from build123d import *

# Parameters (mm, degrees)
F1_W         = 60.96
F1_H         = 78.5
F2_DEPTH     = 21.5
F0_W         = 55.88
F0_H         = 73.5
F3_DEPTH     = 19.5
F4_W         = 78.5
F4_H         = 3
F5_DEPTH     = 2.54
F6_W         = 78.5
F6_H         = 3
F7_DEPTH     = 2.54
F8_W         = 44.0962035209
F8_H         = 7.4383728206
F9_DEPTH     = 2.5
F10_W        = 5.08
F10_H        = 21.59
F11_DEPTH    = 25.4
F12_R        = 1.27
F13_R        = 1.27
F14_DEPTH    = 101.6
F15_R        = 1.27
F16_DEPTH    = 25.4
F17_T1_DEPTH = 2.54
F18_F1_R     = 5.08
F18_T2_DEPTH = 103.9


# Not quite as in the source:
# - a fillet or chamfer that OpenCascade refuses, or shapes differently, is made with other operations: its cross-section is extruded or revolved along the edge and cut away or added


with BuildPart() as f2:
    # F1 (on Top) → F2 (new body)
    with BuildSketch(Plane.XY):
        with Locations((27.94, 36.75)):
            Rectangle(F1_W, F1_H)
    extrude(amount=F2_DEPTH)

    # F0 (on Top) → F3 (cut)
    with BuildSketch(Plane.XY):
        with Locations((27.94, 36.75)):
            Rectangle(F0_W, F0_H)
    extrude(amount=F3_DEPTH, mode=Mode.SUBTRACT)

    # F4 (on face) → F5 (join, through all)
    with BuildSketch(Plane.YZ.offset(58.42)):
        with Locations((36.75, -1.5)):
            Rectangle(F4_W, F4_H)
    extrude(amount=-F5_DEPTH)

    # F6 (on face) → F7 (join, through all)
    with BuildSketch(Plane(origin=(-2.54, 0, 0), x_dir=(0, -1, 0), z_dir=(-1, 0, 0))):
        with Locations((-36.75, -1.5)):
            Rectangle(F6_W, F6_H)
    extrude(amount=-F7_DEPTH)

    # F8 (on face) → F9 (join, through all)
    with BuildSketch(Plane.XZ.offset(2.5)):
        with Locations((27.1060718223, 8.4709739313)):
            Rectangle(F8_W, F8_H)
    extrude(amount=-F9_DEPTH)

    # F10 (on face) → F11 (cut)
    with BuildSketch(Plane(origin=(-2.54, 0, 0), x_dir=(0, -1, 0), z_dir=(-1, 0, 0))):
        with Locations((-2.54, 7.795)):
            Rectangle(F10_W, F10_H)
    extrude(amount=-F11_DEPTH, mode=Mode.SUBTRACT)

    # F12
    f12_edges = [f2.edges().sort_by_distance(p)[0] for p in [
        (-1.27, 0, -3),
        (-1.27, 5.08, -3),
    ]]
    fillet(f12_edges, radius=F12_R)

    # F13 (on face) → F14 (cut)
    with BuildSketch(Plane(origin=(0, 76, 0), x_dir=(-1, 0, 0), z_dir=(0, 1, 0))):
        with Locations((-38.1, 17.955)):
            Circle(F13_R)
    extrude(amount=-F14_DEPTH, mode=Mode.SUBTRACT)

    # F15 (on face) → F16 (cut)
    with BuildSketch(Plane(origin=(-2.54, 0, 0), x_dir=(0, -1, 0), z_dir=(-1, 0, 0))):
        with Locations((-53.768, 11.605)):
            Circle(F15_R)
        with Locations((-19.732, 11.605)):
            Circle(F15_R)
    extrude(amount=-F16_DEPTH, mode=Mode.SUBTRACT)

    # F17: fillet of radius 1.27 on 2 edges, made by hand

    # F17_s2 → F17_t1 (join)
    with BuildSketch(Plane.YZ.offset(-2.54)):
        with BuildLine():
            ThreePointArc((1.2699, 18.5901), (0.3718743879, 18.2181256121), (-0.0001, 17.3201))
            Line((-0.0001, 17.3201), (-0.0255, 17.3201))
            ThreePointArc((-0.0255, 17.3201), (-0.0254, 17.95505), (-0.0254, 18.59))
            Line((-0.0254, 18.59), (0, 18.6154))
            ThreePointArc((0, 18.6154), (0.63495, 18.6154), (1.2699, 18.6155))
            Line((1.2699, 18.6155), (1.2699, 18.5901))
        make_face()
        with BuildLine():
            ThreePointArc((5.0801, 17.3201), (4.7081256121, 18.2181256121), (3.8101, 18.5901))
            Line((3.8101, 18.5901), (3.8101, 18.6155))
            ThreePointArc((3.8101, 18.6155), (4.44505, 18.6154), (5.08, 18.6154))
            Line((5.08, 18.6154), (5.1054, 18.59))
            ThreePointArc((5.1054, 18.59), (5.1054, 17.95505), (5.1055, 17.3201))
            Line((5.1055, 17.3201), (5.0801, 17.3201))
        make_face()
    extrude(amount=F17_T1_DEPTH)

    # F18: fillet of radius 5.08 on 2 edges, made by hand

    # F18_f1
    f18_f1_edges = [f2.edges().sort_by_distance(p)[0] for p in [
        (0, 36.75, 19.5),
    ]]
    fillet(f18_f1_edges, radius=F18_F1_R)

    # F18_s3 → F18_t2 (cut)
    with BuildSketch(Plane.XZ.offset(-88.7)):
        with BuildLine():
            ThreePointArc((-2.54, 16.42), (-1.0521024484, 20.0121024484), (2.54, 21.5))
            Line((2.54, 21.5), (2.54, 21.6016))
            Line((2.54, 21.6016), (-2.6416, 21.6016))
            Line((-2.6416, 21.6016), (-2.6416, 16.42))
            Line((-2.6416, 16.42), (-2.54, 16.42))
        make_face()
    extrude(amount=F18_T2_DEPTH, mode=Mode.SUBTRACT)


solid = f2.part
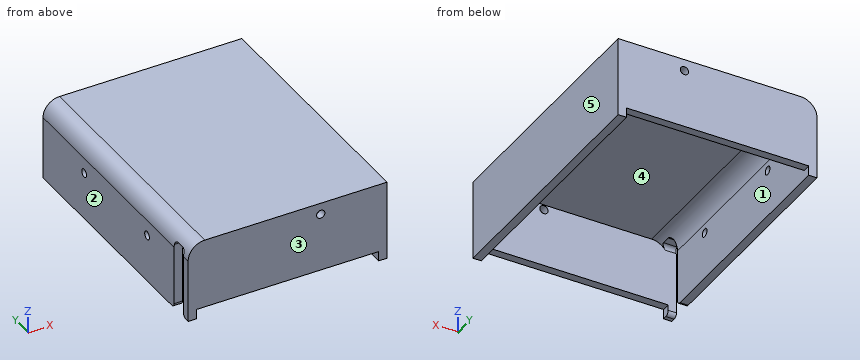
Could you check a few things on this model? Use its own coordinates, in mm. Face numbers are marked on the shaded views. A direction names the side the tool comes from. Give positions to 0.01 mm unless a question says otherwise; leave off trailing zeros. Loops run counter-clockwise (first coordinate to the right, second up) from the corner with the lowest first, then second, coordinate; pieces in that order, holes last. Notation, with made-up numbers: M 68.25,56.25 L 102.25,56.25 A20 cw 102.25,60.25 Z; hole C 5,-34 d9. An arc over 180 degrees is marked long. Answer as a JSON object with one key per item and string values.
Q1. If we mould it in two halves opening along Y, with no side actions, what happens to the marked faces 1, 2 and 3? For each: pulls with the +Y half, pulls with the -Y half, needs draft (parallel to the pull), parting line crosses it, or undercut.
Values found:
{"face 1": "undercut", "face 2": "needs draft", "face 3": "pulls with the -Y half"}
Q2. Suppose I cut it at A-A, the plane x = 38.1. List the corners of the cut face in (y, z) for me (3 decimals).
Values found:
{"outline": "M -2.5,0 L 0,0 L 0,16.685 L -2.5,16.685 Z; M -2.5,19.225 L 0,19.225 L 0,19.5 L 73.5,19.5 L 73.5,19.225 L 76,19.225 L 76,21.5 L -2.5,21.5 Z; M 73.5,0 L 76,0 L 76,16.685 L 73.5,16.685 Z"}
Q3. For the marked faces 4 and 5, which set-ups out of +Z, -Z, +X, -X, +Y, -Y let a thin tool reach every point of the face, with its end or its side?
Values found:
{"face 4": "-Z", "face 5": "+Z, -Z, +X, +Y, -Y"}
Q4. Suppose I cut it at D-D, the plane z = 6.5. List the corners of the cut face in (x, y) for me, plus the area to 3 significant figures.
Values found:
{"outline": "M -2.54,-2.5 L 58.42,-2.5 L 58.42,76 L -2.54,76 L -2.54,5.08 L 0,5.08 L 0,73.5 L 55.88,73.5 L 55.88,0 L -2.54,0 Z", "area": "665 mm²"}
Q5. Suppose I cut it at B-B, the plane y = 48. List the corners of the cut face in (x, z) for me, plus the area to 3 significant figures.
Values found:
{"outline": "M -2.54,-3 L 0,-3 L 0,14.42 A5.08 cw 5.08,19.5 L 55.88,19.5 L 55.88,-3 L 58.42,-3 L 58.42,21.5 L 2.54,21.5 A5.08 ccw -2.54,16.42 Z", "area": "236 mm²"}
Q6. Suppose I cut it at C-C, the plane x = 50. List the corners of the cut face in (y, z) for me.
Values found:
{"outline": "M -2.5,0 L 0,0 L 0,19.5 L 73.5,19.5 L 73.5,0 L 76,0 L 76,21.5 L -2.5,21.5 Z"}
Q7. For P1, Ø1.5, axis at x = 9, y = 32, coming from the -Z side; P2, Ø3, axis at x = 18, y = -1.5, coming from the -Z side; P3, Ø3, axis at x = -1, y = 2.5, coming from the -Z side, each with a flat end and sliding along its axis, tell me the tip position at first contact or that it passes through.
Values found:
{"P1": "stops at z = 19.5", "P2": "stops at z = 0", "P3": "stops at z = 18.56"}
Q8. If I drill on probe 1 along Y at (x, z) = (27, 8.75); probe 2 along X at (y, z) = (52, 1); probe 3 along Z at (x, y) = (38.1, 74) (3 decimals), over which ranges is the centre line in solid material (lowest first)? Write a range as [from, to].
Values found:
{"probe 1": "y = [-2.5, 0], [73.5, 76]", "probe 2": "x = [-2.54, 0], [55.88, 58.42]", "probe 3": "z = [0, 16.685], [19.225, 21.5]"}
